```python
from build123d import *

# Parameters (mm, degrees)
SKETCH1_R                      = 5
BOSS_EXTRUDE1_DEPTH            = 4.25
BOSS_EXTRUDE1_2_DEPTH          = 4.25
SKETCH1_R_2                    = 4.6
BOSS_EXTRUDE1_3_DEPTH          = 4.25
BOSS_EXTRUDE2_DEPTH            = 2.5
BOSS_EXTRUDE3_DEPTH            = 2.75
BOSS_EXTRUDE4_DEPTH            = 4
BOSS_EXTRUDE5_START            = -6.75
SKETCH7_R                      = 3
BOSS_EXTRUDE5_DEPTH            = 6.75
BOSS_EXTRUDE6_DEPTH            = 7
F_2_0_2_DIAMETER_HOLE1_D       = 2
F_2_0_2_DIAMETER_HOLE1_DEPTH   = 1
F_2_0_2_DIAMETER_HOLE1_TIP     = 3.732050808
F_5_2_5_2_DIAMETER_HOLE1_D     = 5.2
F_5_2_5_2_DIAMETER_HOLE1_DEPTH = 41
F_5_2_5_2_DIAMETER_HOLE1_TIP   = 1.562237609


with BuildPart() as part:
    # Sketch1 → Boss-Extrude1 (new body)
    with BuildSketch(Plane.XY):
        with Locations((19.367534606, 34.628988105)):
            Circle(SKETCH1_R)
    extrude(amount=BOSS_EXTRUDE1_DEPTH)



with BuildPart() as body_2:
    # Sketch1 → Boss-Extrude1 2 (new body)
    with BuildSketch(Plane.XY):
        with Locations((-19.466738271, 5.503283448)):
            Circle(SKETCH1_R)
    extrude(amount=BOSS_EXTRUDE1_2_DEPTH)


with BuildPart() as body_3:
    # Sketch1 → Boss-Extrude1 3 (new body)
    with BuildSketch(Plane.XY):
        with Locations((-23.449601832, 51.266135777)):
            Circle(SKETCH1_R_2)
    extrude(amount=BOSS_EXTRUDE1_3_DEPTH)


with BuildPart() as part_1:
    add(part.part)

    add(body_2.part)  # Boss-Extrude2 merges body 2

    add(body_3.part)  # Boss-Extrude2 merges body 3
    # Sketch3 → Boss-Extrude2 (add)
    with BuildSketch(Plane.XY.offset(4.25)):
        with BuildLine():
            Line((-19.895572194, 54.186559261), (-9.131726679, 42.175635572))
            ThreePointArc((-9.131726679, 42.175635572), (-4.375228584, 41.437246463), (-0.389407444, 38.738594493))
            Line((-0.389407444, 38.738594493), (19.051801444, 39.619009405))
            ThreePointArc((19.051801444, 39.619009405), (24.329841267, 35.241778932), (20.275201283, 29.712064148))
            Line((20.275201283, 29.712064148), (1.203848705, 25.836597173))
            ThreePointArc((1.203848705, 25.836597173), (-1.800000005, 22.400000007), (-5.940210923, 20.478552452))
            Line((-5.940210923, 20.478552452), (-14.816024112, 3.667293848))
            ThreePointArc((-14.816024112, 3.667293848), (-21.302727871, 0.852569289), (-24.11745243, 7.339273048))
            Line((-24.11745243, 7.339273048), (-17.566802713, 25.119726319))
            ThreePointArc((-17.566802713, 25.119726319), (-19.323959856, 29.908837282), (-18.731726679, 34.975635572))
            Line((-18.731726679, 34.975635572), (-27.248336676, 48.671985899))
            ThreePointArc((-27.248336676, 48.671985899), (-26.209601832, 54.946135777), (-19.895572194, 54.186559261))
        make_face()
        with BuildLine():
            Line((-8.172170243, 25.06222699), (-7.565580005, 24.253440007))
            ThreePointArc((-7.565580005, 24.253440007), (-5.26029132, 22.888460799), (-2.665020005, 23.553360007))
            ThreePointArc((-2.665020005, 23.553360007), (-1.300040797, 25.858648691), (-1.964940005, 28.453920007))
            Line((-1.964940005, 28.453920007), (-2.571530243, 29.26270699))
            ThreePointArc((-2.571530243, 29.26270699), (-2.337729587, 32.186428603), (-3.486400005, 34.885200007))
            ThreePointArc((-3.486400005, 34.885200007), (-12.085200005, 36.113600007), (-13.313600005, 27.514800007))
            ThreePointArc((-13.313600005, 27.514800007), (-11.044407175, 25.656420412), (-8.172170243, 25.06222699))
        make_face(mode=Mode.SUBTRACT)
    extrude(amount=BOSS_EXTRUDE2_DEPTH)

    # Sketch5 → Boss-Extrude3 (add)
    with BuildSketch(Plane.XY.offset(6.75)):
        with BuildLine():
            Line((8.495879995, 21.742160007), (8.267279995, 22.046960007))
            Line((8.267279995, 22.046960007), (-2.126400462, 35.905200616))
            Line((-2.126400462, 35.905200616), (-5.403000005, 40.274000007))
            Line((-5.403000005, 40.274000007), (-5.479200005, 40.375600007))
            ThreePointArc((-5.479200005, 40.375600007), (-6.963636268, 41.254546165), (-8.634800005, 40.826400007))
            Line((-8.634800005, 40.826400007), (-13.105200005, 37.473600007))
            Line((-13.105200005, 37.473600007), (-17.575600005, 34.120800007))
            ThreePointArc((-17.575600005, 34.120800007), (-18.454546164, 32.636363744), (-18.026400005, 30.965200007))
            Line((-18.026400005, 30.965200007), (-17.950200005, 30.863600007))
            Line((-17.950200005, 30.863600007), (-14.673600388, 26.494800517))
            Line((-14.673600388, 26.494800517), (-4.279920005, 12.636560007))
            Line((-4.279920005, 12.636560007), (-4.051320005, 12.331760007))
            ThreePointArc((-4.051320005, 12.331760007), (-2.566883742, 11.452813848), (-0.895720005, 11.880960007))
            Line((-0.895720005, 11.880960007), (8.045079995, 18.586560007))
            ThreePointArc((8.045079995, 18.586560007), (8.924026154, 20.07099627), (8.495879995, 21.742160007))
        make_face()
        with BuildLine():
            Line((-7.565580005, 24.253440007), (-8.172170243, 25.06222699))
            ThreePointArc((-8.172170243, 25.06222699), (-12.085200005, 36.113600007), (-2.571530243, 29.26270699))
            Line((-2.571530243, 29.26270699), (-1.964940005, 28.453920007))
            ThreePointArc((-1.964940005, 28.453920007), (-2.665020005, 23.553360007), (-7.565580005, 24.253440007))
        make_face(mode=Mode.SUBTRACT)
    extrude(amount=BOSS_EXTRUDE3_DEPTH)

    # Sketch6 → Boss-Extrude4 (add)
    with BuildSketch(Plane.XY.offset(9.5)):
        with BuildLine():
            Line((-8.634800005, 40.826400007), (-13.105200005, 37.473600007))
            Line((-13.105200005, 37.473600007), (-17.575600005, 34.120800007))
            ThreePointArc((-17.575600005, 34.120800007), (-18.454546164, 32.636363744), (-18.026400005, 30.965200007))
            Line((-18.026400005, 30.965200007), (-17.950200005, 30.863600007))
            Line((-17.950200005, 30.863600007), (-14.673600388, 26.494800517))
            Line((-14.673600388, 26.494800517), (-4.279920005, 12.636560007))
            Line((-4.279920005, 12.636560007), (-4.051320005, 12.331760007))
            ThreePointArc((-4.051320005, 12.331760007), (-2.566883742, 11.452813848), (-0.895720005, 11.880960007))
            Line((-0.895720005, 11.880960007), (8.045079995, 18.586560007))
            ThreePointArc((8.045079995, 18.586560007), (8.924026154, 20.07099627), (8.495879995, 21.742160007))
            Line((8.495879995, 21.742160007), (8.267279995, 22.046960007))
            Line((8.267279995, 22.046960007), (-2.126400462, 35.905200616))
            Line((-2.126400462, 35.905200616), (-5.403000005, 40.274000007))
            Line((-5.403000005, 40.274000007), (-5.479200005, 40.375600007))
            ThreePointArc((-5.479200005, 40.375600007), (-6.963636268, 41.254546165), (-8.634800005, 40.826400007))
        make_face()
        with BuildLine():
            Line((6.907279995, 21.026960007), (-3.486400462, 34.885200616))
            Line((-3.486400462, 34.885200616), (-6.763000005, 39.254000007))
            Line((-6.763000005, 39.254000007), (-6.839200005, 39.355600007))
            ThreePointArc((-6.839200005, 39.355600007), (-7.204052574, 39.571632026), (-7.614800005, 39.466400007))
            Line((-7.614800005, 39.466400007), (-12.085200005, 36.113600007))
            Line((-12.085200005, 36.113600007), (-16.555600005, 32.760800007))
            ThreePointArc((-16.555600005, 32.760800007), (-16.771632024, 32.395947438), (-16.666400005, 31.985200007))
            Line((-16.666400005, 31.985200007), (-16.590200005, 31.883600007))
            Line((-16.590200005, 31.883600007), (-13.313600388, 27.514800517))
            Line((-13.313600388, 27.514800517), (-2.919920005, 13.656560007))
            Line((-2.919920005, 13.656560007), (-2.691320005, 13.351760007))
            ThreePointArc((-2.691320005, 13.351760007), (-2.326467436, 13.135727987), (-1.915720005, 13.240960007))
            Line((-1.915720005, 13.240960007), (7.025079995, 19.946560007))
            ThreePointArc((7.025079995, 19.946560007), (7.241112015, 20.311412575), (7.135879995, 20.722160007))
            Line((7.135879995, 20.722160007), (6.907279995, 21.026960007))
        make_face(mode=Mode.SUBTRACT)
    extrude(amount=BOSS_EXTRUDE4_DEPTH)

    # Sketch7 → Boss-Extrude5 (add)
    with BuildSketch(Plane.XY.offset(13.5).offset(BOSS_EXTRUDE5_START)):
        with Locations((-12.956760005, 37.275680007)):
            Circle(SKETCH7_R)
        with Locations((3.426239995, 15.431680007)):
            Circle(SKETCH7_R)
    extrude(amount=BOSS_EXTRUDE5_DEPTH)

    # Sketch8 → Boss-Extrude6 (add)
    with BuildSketch(Plane.XY.offset(13.5)):
        Polygon((-16.666400005, 31.985200007), (-18.026400005, 30.965200007), (-4.051320005, 12.331760007), (-2.691320005, 13.351760007), align=None)
    extrude(amount=BOSS_EXTRUDE6_DEPTH)

    # Ø2.0 (2) Diameter Hole1
    with Locations(Plane.XY.offset(13.5)):
        with Locations((-12.956760005, 37.275680007), (3.426239995, 15.431680007)):
            Hole(F_2_0_2_DIAMETER_HOLE1_D / 2, depth=F_2_0_2_DIAMETER_HOLE1_DEPTH)
            with Locations((0, 0, -(F_2_0_2_DIAMETER_HOLE1_DEPTH + F_2_0_2_DIAMETER_HOLE1_TIP / 2))):  # 30° drill point
                Cone(0, F_2_0_2_DIAMETER_HOLE1_D / 2, F_2_0_2_DIAMETER_HOLE1_TIP, mode=Mode.SUBTRACT)

    # Ø5.2 (5.2) Diameter Hole1
    with Locations(Plane(origin=(-108.726431202, 76.790635104, -28), x_dir=(-0.6000000000000003, 0.7999999999999998, 4.198929075555247e-15), z_dir=(0, 0, -1))):
        with Locations((-110.585697084, 28.635343351), (-71.585697084, 52.906763899), (-110.585697084, 77.178184447)):
            Hole(F_5_2_5_2_DIAMETER_HOLE1_D / 2, depth=F_5_2_5_2_DIAMETER_HOLE1_DEPTH)
            with Locations((0, 0, -(F_5_2_5_2_DIAMETER_HOLE1_DEPTH + F_5_2_5_2_DIAMETER_HOLE1_TIP / 2))):  # 118° drill point
                Cone(0, F_5_2_5_2_DIAMETER_HOLE1_D / 2, F_5_2_5_2_DIAMETER_HOLE1_TIP, mode=Mode.SUBTRACT)


solid = part_1.part
```
The listing builds one solid part. Answer for the finished solid, in the listing's coordinates (mm). A direction names the side the tool comes from. Give positions to 0.01 mm unless a question says otherwise; leave off trailing zeros. Order: outer loops, then holes, each group sorted by start corner. A loop starts at its lowest first (then second) coordinate and runs counter-clockwise, first axis right, second up. Notation, with made-up numbers: M 67.5,7.25 L 86.5,7.25 A4 cw 86.5,13.25 Z; hole C 12.5,0 d5. An arc over 180 degrees is marked long. Put each result on its own line as item: value. Start each with the question number.
Item 1: The part is cut by section A-A, the plane z = 5.25. Determine the outline of the cut face in (x, y).
Item 2: The part is cut by section B-B, the plane x = 18. Determine the outline of the cut face in (y, z).
Item 3: Which of the six approach directions +Z, -Z, +X, -X, +Y, -Y give full straight-line access (tool end or side, diameter ignored) to faces 5 (the face through (-17.34, 31.48, 16.95)), 6 (the face through (-15.354, 33.662, 11.472)), 7 (the face through (-9.66, 40.06, 10.08))?
Item 4: Find the intervals of material crossed by line 1 along Z through (x, y) = (20, 31); line 2 along Y through (x, z) = (-18.5, 1); line 3 along Z through (x, y) = (-2, 23), in increasing order.
Item 5: Flat-ended cylindrical pins translate along their axes: P1, Ø12, axis at x = 3, y = 17.5, coming from the -Z side; P2, Ø2, axis at y = 34, z = 10.5, coming from the -X side; P3, Ø8, axis at x = 6, y = 30.5, coming from the +Z side. Find the tip coordinate at first contact, or state that the pin passes through.
Item 6: The part is cut by section C-C, the plane y = 9. Determine the outline of the cut face in (x, z).
Item 7: For a pull along X with two mould halves and no side action, classify faces 1 (the face through (-3.381, 12.835, 16.951)), 2 (the face through (-17, 3, 0)), 3 (the face through (5.176, 12.995, 10.078)), 4 (the face through (-20.888, 16.105, 5.482)) as +X half, -X half, draft (parallel to the pull), parting line (faces both ways), or undercut.
Item 8: The part is cut by section D-D, the plane z = 14.75. Determine the outline of the cut face in (x, y), and give its area (3 significant figures).
Answer key:
1. outline: M -27.25,48.67 L -18.73,34.98 A11 ccw -17.57,25.12 L -24.12,7.34 A5 ccw -14.82,3.67 L -5.94,20.48 A11 ccw 1.2,25.84 L 20.28,29.71 A5 ccw 19.05,39.62 L -0.39,38.74 A11 ccw -9.13,42.18 L -19.9,54.19 A4.6 ccw Z; hole C -23.45,51.27 d5.2; hole C -19.47,5.5 d5.2; hole M -8.17,25.06 L -7.57,24.25 A3.5 ccw -1.96,28.45 L -2.57,29.26 A6.14 ccw long Z; hole C 19.37,34.63 d5.2
2. outline: M 29.25,4.25 L 29.82,4.25 L 29.82,0 L 32.42,0 L 32.42,6.75 L 29.25,6.75 Z; M 36.84,0 L 39.44,0 L 39.44,4.25 L 39.57,4.25 L 39.57,6.75 L 36.84,6.75 Z
3. face 5: +Z, -X, +Y
3. face 6: +Z
3. face 7: +Z, +Y
4. line 1: z = 0 to 6.75
4. line 2: y = 0.6 to 3.09, 7.92 to 10.41
4. line 3: z = 4.25 to 9.5
5. P1: stops at z = 6.75
5. P2: stops at x = -18.37
5. P3: stops at z = 13.5
6. outline: M -23.51,4.25 L -23.04,4.25 L -23.04,0 L -15.89,0 L -15.89,4.25 L -12,4.25 L -12,6.75 L -23.51,6.75 Z
7. face 1: +X half
7. face 2: draft
7. face 3: undercut
7. face 4: -X half
8. outline: M -18.03,30.97 L -4.05,12.33 L -2.69,13.35 L -16.67,31.99 Z
8. area: 39.6 mm²
